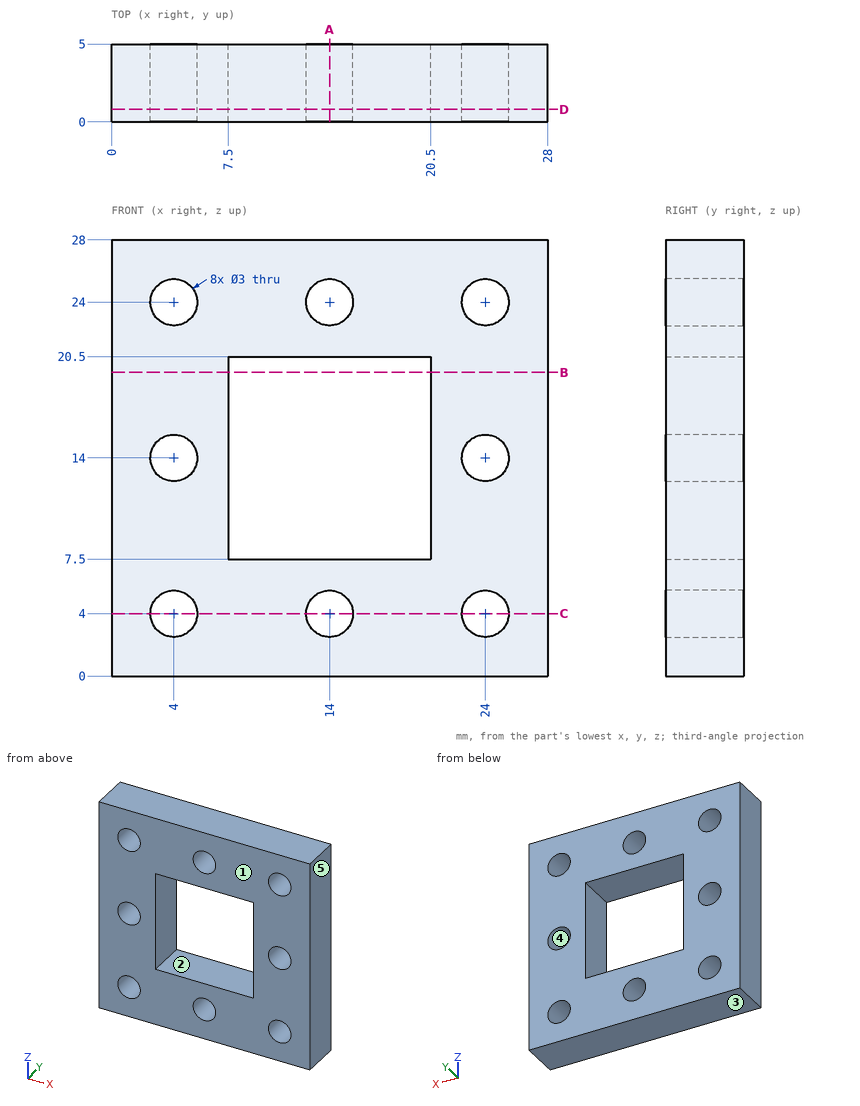
Source: three-view drawing plus pictorial views. Frame: mm from the lowest corner of the part. A direction names the side the tool comes from. Give positions to 0.01 mm unless a question says otherwise; leave off trailing zeros. Loops run counter-clockwise (first coordinate to the right, second up) from the corner with the lowest first, then second, coordinate; pieces in that order, holes last. Notation, with made-up numbers: (-24.75, 23) -> (5.25, 23) arc R8 ccw to (5.25, 28) -> close; hole circle Ø8 at (22.5, 4.5). An arc over 180 degrees is marked (long way). Put each result on its own line as item: value. Start each with the question number.
1) Draft query along X for the marked faces 3, 4 and 5. Return one class per face: released by +X, released by -X, zero draft, split by the parting line, or undercut.
2) Cut plane A-A (x = 14). Return loops of the section in (y, z).
3) Cut plane D-D (y = 0.8). State how many separate pieces and enclosed holes the cut face has, then the cut area to 3 significant figures.
4) Cut plane C-C (z = 4). Return loops of the section in (x, y).
5) Contact query for a flat-ended pin moving along its axis: P1, Ø1.8, axis at x = 24, z = 24, coming from the -Y side. Output: stop coordinate, or through.
6) Cut plane B-B (z = 19.5). Return loops of the section in (x, y).
7) Reachability of the marked faces 1 and 2 from +Z, -Z, +X, -X, +Y, -Y: full face, straight path, thin tool, end or side. Return the list, or none.
8) Material intervals for probe 1 along X at (y, z) = (3.25, 14); probe 2 along X at (y, z) = (3.6, 24); probe 3 along X at (y, z) = (1.4, 9.5), sorted ascending.
Results are:
1. face 3: zero draft
1. face 4: undercut
1. face 5: released by +X
2. outline: (0, 0) -> (5, 0) -> (5, 2.5) -> (0, 2.5) -> close; (0, 5.5) -> (5, 5.5) -> (5, 7.5) -> (0, 7.5) -> close; (0, 20.5) -> (5, 20.5) -> (5, 22.5) -> (0, 22.5) -> close; (0, 25.5) -> (5, 25.5) -> (5, 28) -> (0, 28) -> close
3. separate pieces: 1
3. enclosed holes: 9
3. area: 558 mm2
4. outline: (0, 0) -> (2.5, 0) -> (2.5, 5) -> (0, 5) -> close; (5.5, 0) -> (12.5, 0) -> (12.5, 5) -> (5.5, 5) -> close; (15.5, 0) -> (22.5, 0) -> (22.5, 5) -> (15.5, 5) -> close; (25.5, 0) -> (28, 0) -> (28, 5) -> (25.5, 5) -> close
5. P1: passes through
6. outline: (0, 0) -> (7.5, 0) -> (7.5, 5) -> (0, 5) -> close; (20.5, 0) -> (28, 0) -> (28, 5) -> (20.5, 5) -> close
7. face 1: +Z, -Z, +X, -X, -Y
7. face 2: +Y, -Y
8. probe 1: x = 0 to 2.5, 5.5 to 7.5, 20.5 to 22.5, 25.5 to 28
8. probe 2: x = 0 to 2.5, 5.5 to 12.5, 15.5 to 22.5, 25.5 to 28
8. probe 3: x = 0 to 7.5, 20.5 to 28
